Build history of the part. All positions in model axes, mm. A direction names the side the tool comes from. Give positions to 0.01 mm unless a question says otherwise; leave off trailing zeros. Order: outer loops, then holes, each group sorted by start corner. A loop starts at its lowest first (then second) coordinate and runs counter-clockwise, first axis right, second up. Notation, with made-up numbers: (61, 28.5) -> (97, 28.5) arc R20 ccw to (97, 67.5) -> close; hole circle Ø1 at (28, 16). An arc over 180 degrees is marked (long way). One line per item, written item: value. Start each with the question number.
(1) Saw through at C-C on z = 6.5. Give the cut face in (x, y).
(2) Saw through at D-D on x = -36. Give the cut face in (y, z).
(3) Saw through at B-B on y = 5. Give the cut face in (x, z), plus the area to 3 significant figures.
(4) Probe line 1 (Y direction, x = 25, z = 7); line 2 (X direction, y = -5.25, z = 5); line 3 (Z direction, x = -42.5, y = 0). List the from-to ranges inside material, lowest first.
(5) Two-plate mould, pull along Y, no slides. Class faces 1 (the flat face through (-30, 0, 0)), 2 (the flat face through (0, 0, 15)), 3 (the flat face through (0, 15, 0)): +Y half, -Y half, draft (parallel to the pull), parting line (faces both ways), or undercut.
(6) Saw through at A-A on x = 25. Give the cut face in (y, z), plus the area to 3 significant figures.
(7) Which spindle directions (+Z, -Z, +X, -X, +Y, -Y) get a long thin tool onto all of the face, cutting with end or side? Do faces 4 (the flat face through (-30, -12, 12)), 5 (the flat face through (-30, 12, -11)), 6 (the flat face through (-30, -11, -12)), 7 (the flat face through (-30, 12, 11)), 8 (the cylindrical face through (-42.325, 14.985, -0.66)). Say none if no direction does.
(8) Pin check, flat tip, straight feed: pin 1 (5 mm diameter, centred on y = -2, z = -2.5, fed in from -X). Stop position of the tip, or through.
Solid Edge part; units mm, degrees
sketch "Sketch1" plane through (0, 0, 0) normal (0, 0, 1) x (1, 0, 0)
  line L0 (-30, -15) -> (30, -15)
  line L1 (30, -15) -> (30, 15)
  line L2 (30, 15) -> (-30, 15)
  line L3 (-30, 15) -> (-30, -15)
  circle A0 centre (25, 5) radius 2.5
  circle A1 centre (25, -5) radius 2.5
extrude "Protrusion1" add sketch "Sketch1" along normal mid plane 30
sketch "Sketch2" plane through (-30, 0, 0) normal (-1, 0, 0) x (0, -1, 0)
  circle A0 centre (0, 0) radius 15
  circle A1 centre (0, 0) radius 12.5
extrude "ExtrudedProtrusion_2" add sketch "Sketch2" along normal mid plane 50
properties material "Steel - Stainless:1.4404 , X2CrNiMo17-12-2"
Results below:
1. outline: (-55, -13.52) -> (-30, -13.52) -> (-30, -15) -> (30, -15) -> (30, 15) -> (-30, 15) -> (-30, 13.52) -> (-55, 13.52) -> (-55, 10.68) -> (-30, 10.68) -> (-30, -10.68) -> (-55, -10.68) -> close; hole circle Ø5 at (25, -5); hole circle Ø5 at (25, 5)
2. outline: circle Ø30 at (0, 0); hole circle Ø25 at (0, 0)
3. outline: (-55, -14.14) -> (-30, -14.14) -> (-30, -15) -> (22.5, -15) -> (22.5, 15) -> (-30, 15) -> (-30, 14.14) -> (-55, 14.14) -> (-55, 11.46) -> (-30, 11.46) -> (-30, -11.46) -> (-55, -11.46) -> close; (27.5, -15) -> (30, -15) -> (30, 15) -> (27.5, 15) -> close
3. area: 1,780 mm²
4. line 1: y = -15 to -7.5, -2.5 to 2.5, 7.5 to 15
4. line 2: x = -30 to 22.51, 27.49 to 30
4. line 3: z = -15 to -12.5, 12.5 to 15
5. face 1: undercut
5. face 2: draft
5. face 3: +Y half
6. outline: (-15, -15) -> (-7.5, -15) -> (-7.5, 15) -> (-15, 15) -> close; (-2.5, -15) -> (2.5, -15) -> (2.5, 15) -> (-2.5, 15) -> close; (7.5, -15) -> (15, -15) -> (15, 15) -> (7.5, 15) -> close
6. area: 600 mm²
7. face 4: +Z, -X, -Y
7. face 5: -Z, -X, +Y
7. face 6: -Z, -X, -Y
7. face 7: +Z, -X, +Y
7. face 8: -X
8. pin 1: stops at x = -30
